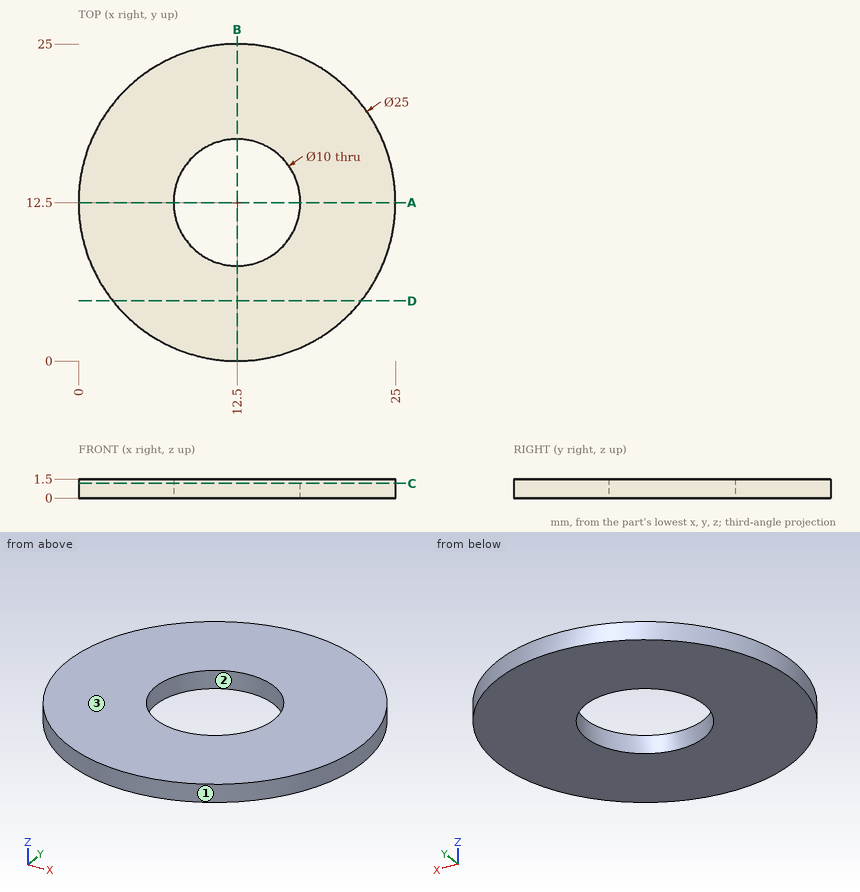
Can you work these out from the drawing? Everything is in mm from the part's minimum corner. Give positions to 0.01 mm unless a question says otherwise; leave off trailing zeros. Loops run counter-clockwise (first coordinate to the right, second up) from the corner with the lowest first, then second, coordinate; pieces in that order, holes last. Notation, with made-up numbers: (36.5, 38.25) -> (57.5, 38.25) arc R29 cw to (57.5, 58.25) -> close; hole circle Ø8 at (21.5, -13.5). An arc over 180 degrees is marked (long way). Return JSON: item names as keys, results as strings.
Item 1: If we section it at C-C on z = 1.15: List the corners of the cut face in (x, y) for me, plus the area to 3 significant figures.
Geometry results:
{"outline": "circle Ø25 at (12.5, 12.5); hole circle Ø10 at (12.5, 12.5)", "area": "412 mm²"}
Item 2: I need wall thicknesses on L1, parallel to Y at x = 12.5, z = 0.5; L2, parallel to X at y = 14.75, z = 0.5; L3, parallel to X at y = 12, z = 0.5. Which ranges of each line are inside material? Lowest first, please. Write a range as from..to.
Geometry results:
{"L1": "y = 0..7.5, 17.5..25", "L2": "x = 0.2..8.03, 16.97..24.8", "L3": "x = 0.01..7.53, 17.47..24.99"}
Item 3: If we section it at D-D on y = 4.75: List the corners of the cut face in (x, z) for me.
Geometry results:
{"outline": "(2.69, 0) -> (22.31, 0) -> (22.31, 1.5) -> (2.69, 1.5) -> close"}
Item 4: If we section it at A-A on y = 12.5: List the corners of the cut face in (x, z) for me.
Geometry results:
{"outline": "(0, 0) -> (7.5, 0) -> (7.5, 1.5) -> (0, 1.5) -> close; (17.5, 0) -> (25, 0) -> (25, 1.5) -> (17.5, 1.5) -> close"}
Item 5: We'd pull the mould along Y, two halves only. Please class the marked faces 1, 2 and 3: +Y half, -Y half, draft (parallel to the pull), parting line (faces both ways), or undercut.
Geometry results:
{"face 1": "parting line", "face 2": "undercut", "face 3": "draft"}
